Could you check a few things on this drawing? It's one solid part, dimensions in mm from its lowest x, y, z. Give positions to 0.01 mm unless a question says otherwise; leave off trailing zeros. Order: outer loops, then holes, each group sorted by start corner. A loop starts at its lowest first (then second) coordinate and runs counter-clockwise, first axis right, second up.
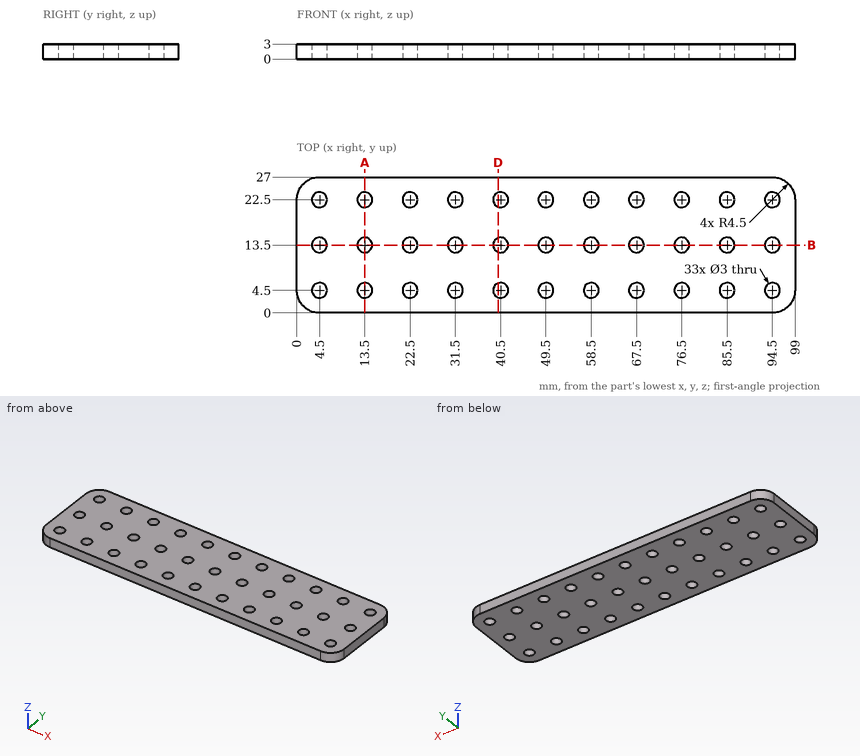
Q1. I need wall thicknesses on L1, parallel to Y at x = 4.5, z = 0.25; L2, parallel to Y at x = 4, z = 1.75. Which ranges of each line are inside material? Lowest first, please.
Filled sheet:
L1: y = 0 to 3, 6 to 12, 15 to 21, 24 to 27
L2: y = 0.03 to 3.09, 5.91 to 12.09, 14.91 to 21.09, 23.91 to 26.97
Q2. If we section it at A-A on x = 13.5: List the corners of the cut face in (y, z) for me.
Filled sheet:
outline: (0, 0) - (3, 0) - (3, 3) - (0, 3) - close; (6, 0) - (12, 0) - (12, 3) - (6, 3) - close; (15, 0) - (21, 0) - (21, 3) - (15, 3) - close; (24, 0) - (27, 0) - (27, 3) - (24, 3) - close
Q3. I'm going to push a flat-ended pin straight in: P1, Ø3.5, axis at x = 58.5, y = 22.5, coming from the +Z side. Where does the tip first touch, or does it pass through?
Filled sheet:
P1: stops at z = 3
Q4. If we section it at B-B on y = 13.5: Give the number of separate pieces and of enclosed holes in the cut face, plus the area to 3 significant figures.
Filled sheet:
separate pieces: 12
enclosed holes: 0
area: 198 mm2
Q5. If we section it at D-D on x = 40: List the corners of the cut face in (y, z) for me.
Filled sheet:
outline: (0, 0) - (3.09, 0) - (3.09, 3) - (0, 3) - close; (5.91, 0) - (12.09, 0) - (12.09, 3) - (5.91, 3) - close; (14.91, 0) - (21.09, 0) - (21.09, 3) - (14.91, 3) - close; (23.91, 0) - (27, 0) - (27, 3) - (23.91, 3) - close
